Verification items for the finished model (mm, model axes). Face numbers are marked on the shaded views. Coordinates: 2 decimals unless noted, no trailing zeros. Write each loop counter-clockwise with the first axis right and the second up, starting at its lowest first coordinate (ties: lowest second). Pieces come first, ordered by that corner, then holes. Notation, with made-up numbers: M 29.25,63.25 L 52.25,63.25 A17 cw 52.25,67.25 Z; hole C 25.5,76 d3. An arc over 180 degrees is marked long. Answer in a Markdown table with one row per item.
from build123d import *

# Parameters (mm, degrees)
F0_W     = 56
F0_H     = 45
F0_W_2   = 52
F0_H_2   = 41
F1_DEPTH = 6
F0_W_3   = 88.9
F0_H_3   = 63.5
F2_DEPTH = 2
F3_DEPTH = 2


with BuildPart() as f1:
    # F0 (on Top) → F1 (new body)
    with BuildSketch(Plane.XY):
        with Locations((44.45, 31.75)):
            Rectangle(F0_W, F0_H)
        with Locations((44.45, 31.75)):
            Rectangle(F0_W_2, F0_H_2, mode=Mode.SUBTRACT)
    extrude(amount=F1_DEPTH)

    # F0 (on Top) → F2 (join)
    with BuildSketch(Plane.XY):
        with Locations((44.45, 31.75)):
            Rectangle(F0_W_3, F0_H_3)
        with Locations((44.45, 31.75)):
            Rectangle(F0_W, F0_H, mode=Mode.SUBTRACT)
    extrude(amount=F2_DEPTH)

    # F0 (on Top) → F3 (join)
    with BuildSketch(Plane.XY):
        with Locations((44.45, 31.75)):
            Rectangle(F0_W_2, F0_H_2)
    extrude(amount=F3_DEPTH)

    # F4: F1 across plane


with BuildPart() as f1_1:
    add(f1.part)
    add(f1.part.mirror(Plane.YZ))


solid = f1_1.part
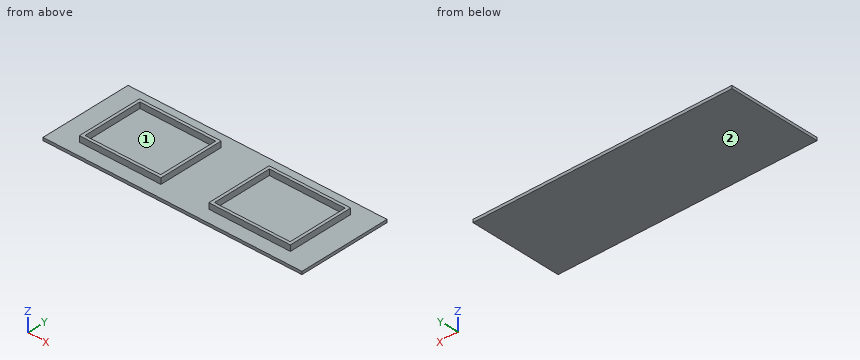
1) Sectioned sample at B-B (x = 30). Record the cut outline in (y, z).
Response values:
| item | result |
|---|---|
| outline | M 0,0 L 63.5,0 L 63.5,2 L 54.25,2 L 54.25,6 L 52.25,6 L 52.25,2 L 11.25,2 L 11.25,6 L 9.25,6 L 9.25,2 L 0,2 Z |
2) Depth check by flat-ended pin: pin 1 (2 mm diameter, centred on x = 35.5, z = 3.5, fed in from -Y); pin 2 (2 mm diameter, centred on x = -4, y = 7, fed in from +Z); pin 3 (2 mm diameter, centred on y = 29.5, z = 4, fed in from -X). Enter the tip coordinate at first touch or a pass-through.
Response values:
| item | result |
|---|---|
| pin 1 | stops at y = 9.25 |
| pin 2 | stops at z = 2 |
| pin 3 | stops at x = -72.45 |
3) Sectioned sample at D-D (x = 78.5). Record the cut outline in (y, z), then the cut area to 3 significant figures.
Response values:
| item | result |
|---|---|
| outline | M 0,0 L 63.5,0 L 63.5,2 L 0,2 Z |
| area | 127 mm² |
4) Sectioned sample at C-C (y = 18). Record the cut outline in (x, z), then the cut area to 3 significant figures.
Response values:
| item | result |
|---|---|
| outline | M -88.9,0 L 88.9,0 L 88.9,2 L 72.45,2 L 72.45,6 L 70.45,6 L 70.45,2 L 18.45,2 L 18.45,6 L 16.45,6 L 16.45,2 L -16.45,2 L -16.45,6 L -18.45,6 L -18.45,2 L -70.45,2 L -70.45,6 L -72.45,6 L -72.45,2 L -88.9,2 Z |
| area | 388 mm² |
5) Release check for a two-part mould opening along X. For the marked faces 1 and 2 record: +X half, -X half, draft (parallel to the pull), parting line (faces both ways), or undercut.
Response values:
| item | result |
|---|---|
| face 1 | undercut |
| face 2 | draft |
6) Thickness scan on L1, parallel to X at y = 13.5, z = 5.65; L2, parallel to Y at x = -55, z = 3.9; L3, parallel to X at y = 10.5, z = 4.3. Record the ranges inside material, lowest first. Write a range as [from, to].
Response values:
| item | result |
|---|---|
| L1 | x = [-72.45, -70.45], [-18.45, -16.45], [16.45, 18.45], [70.45, 72.45] |
| L2 | y = [9.25, 11.25], [52.25, 54.25] |
| L3 | x = [-72.45, -16.45], [16.45, 72.45] |
7) Sectioned sample at A-A (z = 3.5). Record the cut outline in (x, y).
Response values:
| item | result |
|---|---|
| outline | M -72.45,9.25 L -16.45,9.25 L -16.45,54.25 L -72.45,54.25 Z; M 16.45,9.25 L 72.45,9.25 L 72.45,54.25 L 16.45,54.25 Z; hole M -70.45,11.25 L -18.45,11.25 L -18.45,52.25 L -70.45,52.25 Z; hole M 18.45,11.25 L 70.45,11.25 L 70.45,52.25 L 18.45,52.25 Z |
